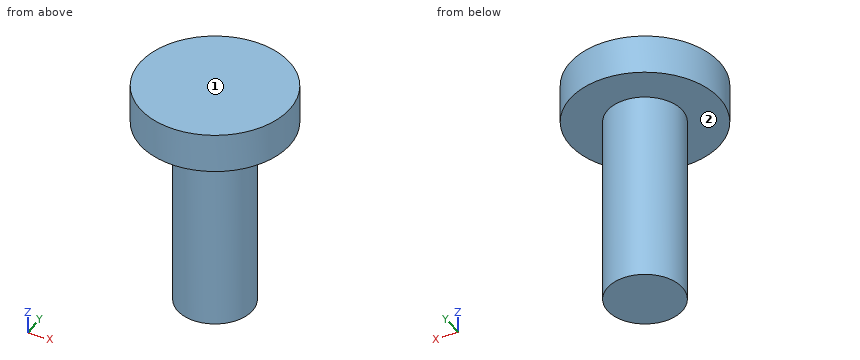
from build123d import *

# Parameters (mm, degrees)
SKETCH039_R  = 1.9
PAD015_DEPTH = 6
SKETCH040_R  = 3.8
PAD016_DEPTH = 2
SKETCH049_R  = 1.9
PAD023_DEPTH = 3.8


with BuildPart() as part:
    # Sketch039 (on Face1 of CopyPocket020) → Pad015 (new body)
    with BuildSketch(Plane.XY.offset(14)):
        with Locations((36, 0)):
            Circle(SKETCH039_R)
    extrude(amount=PAD015_DEPTH)

    # Sketch040 (on Face3 of Pad015) → Pad016 (join)
    with BuildSketch(Plane.XY.offset(20)):
        with Locations((36, 0)):
            Circle(SKETCH040_R)
    extrude(amount=PAD016_DEPTH)

    # Sketch049 (on Face1 of Pad016) → Pad023 (join)
    with BuildSketch(Plane(origin=(0, 0, 14), x_dir=(1, 0, 0), z_dir=(0, 0, -1))):
        with Locations((36, 0)):
            Circle(SKETCH049_R)
    extrude(amount=PAD023_DEPTH)


solid = part.part
Geometry: final body of the model. Coordinates: model frame, mm. Face numbers are marked on the shaded views. A direction names the side the tool comes from. Round coordinates to 2 decimals unless told otherwise and drop trailing zeros. Loops run counter-clockwise (first coordinate to the right, second up) from the corner with the lowest first, then second, coordinate; pieces in that order, holes last. Notation, with made-up numbers: (5, -1.5) - (32, -1.5) arc R23 ccw to (32, 16.5) - close; hole circle Ø10 at (73.5, 28.5). An arc over 180 degrees is marked (long way). Write each question's results on one line, items separated by ' | '. Start each with the question number.
1) Cut plane D-D on y = -3. Return loops of the section in (x, z), then the cut area to 3 significant figures.
2) Cut plane C-C on z = 15.25. Return loops of the section in (x, y).
3) Cut plane B-B on y = 0.5. Return loops of the section in (x, z), then the cut area to 3 significant figures.
4) First-contact query: P1, Ø2, axis at x = 37, z = 11.5, coming from the +Y side. Flat tip, straight axial feed; report the tip coordinate or a pass-through.
5) Line query: probe 1 along Z at (x, y) = (38, -0.75); probe 2 along X at (y, z) = (2.25, 21.5); probe 3 along Y at (x, z) = (34.75, 13.5). Output: solid intervals per line, ascending. Write a range as [from, to].
6) Cut plane A-A on x = 36. Return loops of the section in (y, z).
7) Access query for the marked faces 1 and 2. Directions: +Z, -Z, +X, -X, +Y, -Y. A direction counts if a zero-diameter tool reaches every point of the face in a straight line with its end or side. Return the directions, or none.
Verdict:
1) outline: (33.67, 20) - (38.33, 20) - (38.33, 22) - (33.67, 22) - close | area: 9.33 mm2
2) outline: circle Ø3.8 at (36, 0)
3) outline: (32.23, 20) - (34.17, 20) - (34.17, 10.2) - (37.83, 10.2) - (37.83, 20) - (39.77, 20) - (39.77, 22) - (32.23, 22) - close | area: 51.0 mm2
4) P1: stops at y = 1.9
5) probe 1: z = [20, 22] | probe 2: x = [32.94, 39.06] | probe 3: y = [-1.43, 1.43]
6) outline: (-3.8, 20) - (-1.9, 20) - (-1.9, 10.2) - (1.9, 10.2) - (1.9, 20) - (3.8, 20) - (3.8, 22) - (-3.8, 22) - close
7) face 1: +Z, +X, -X, +Y, -Y | face 2: -Z
